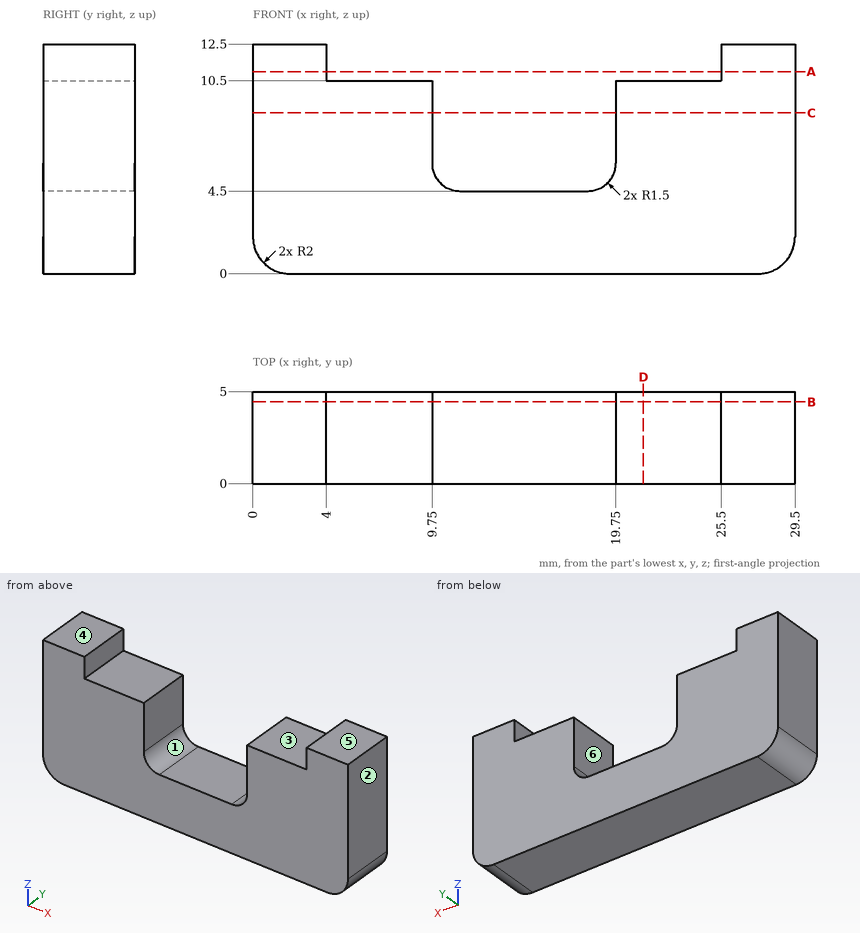
Geometry check sheet. Reference: drawing and pictorial views, mm from the part's lowest x, y, z. A direction names the side the tool comes from. Give positions to 0.01 mm unless a question says otherwise; leave off trailing zeros. Loops run counter-clockwise (first coordinate to the right, second up) from the corner with the lowest first, then second, coordinate; pieces in that order, holes last.
1. Section check B-B, the plane y = 4.45. Enter the section's corners in (x, z).
2. Go/stop test with a flat-tipped pin: pin 1 Ø2.5 at (x, y) = (23, 1.5) entering from +Z. Record where the tip stops, or that it passes through.
3. Section check D-D, the plane x = 21.25. Enter the section's corners in (y, z).
4. Section check A-A, the plane z = 11. Enter the section's corners in (x, y), then the cut area to 3 significant figures.
5. Set-up check for the marked faces 5 and 6: record each of +Z, -Z, +X, -X, +Y, -Y from which the full face is reachable in a straight line by a thin tool's end or side.
6. Section check C-C, the plane z = 8.75. Enter the section's corners in (x, y), then the cut area to 3 significant figures.
7. Mould release check, pull along X, two halves, no side actions. Record for the marked faces 1, 2, 3 and 4: released by +X, released by -X, zero draft, split by the parting line, or undercut.
8. Thickness scan on line 1 (X direction, y = 2.85, z = 10.75); line 2 (X direction, y = 0.2, z = 8); line 3 (Z direction, x = 13, y = 1.75). Record the ranges inside material, lowest first.
Geometry says:
1. outline: (0, 2) arc R2 ccw to (2, 0) - (27.5, 0) arc R2 ccw to (29.5, 2) - (29.5, 12.5) - (25.5, 12.5) - (25.5, 10.5) - (19.75, 10.5) - (19.75, 6) arc R1.5 cw to (18.25, 4.5) - (11.25, 4.5) arc R1.5 cw to (9.75, 6) - (9.75, 10.5) - (4, 10.5) - (4, 12.5) - (0, 12.5) - close
2. pin 1: stops at z = 10.5
3. outline: (0, 0) - (5, 0) - (5, 10.5) - (0, 10.5) - close
4. outline: (0, 0) - (4, 0) - (4, 5) - (0, 5) - close; (25.5, 0) - (29.5, 0) - (29.5, 5) - (25.5, 5) - close
4. area: 40.0 mm2
5. face 5: +Z, +X, -X, +Y, -Y
5. face 6: +Z, +Y, -Y
6. outline: (0, 0) - (9.75, 0) - (9.75, 5) - (0, 5) - close; (19.75, 0) - (29.5, 0) - (29.5, 5) - (19.75, 5) - close
6. area: 97.5 mm2
7. face 1: undercut
7. face 2: released by +X
7. face 3: undercut
7. face 4: zero draft
8. line 1: x = 0 to 4, 25.5 to 29.5
8. line 2: x = 0 to 9.75, 19.75 to 29.5
8. line 3: z = 0 to 4.5
